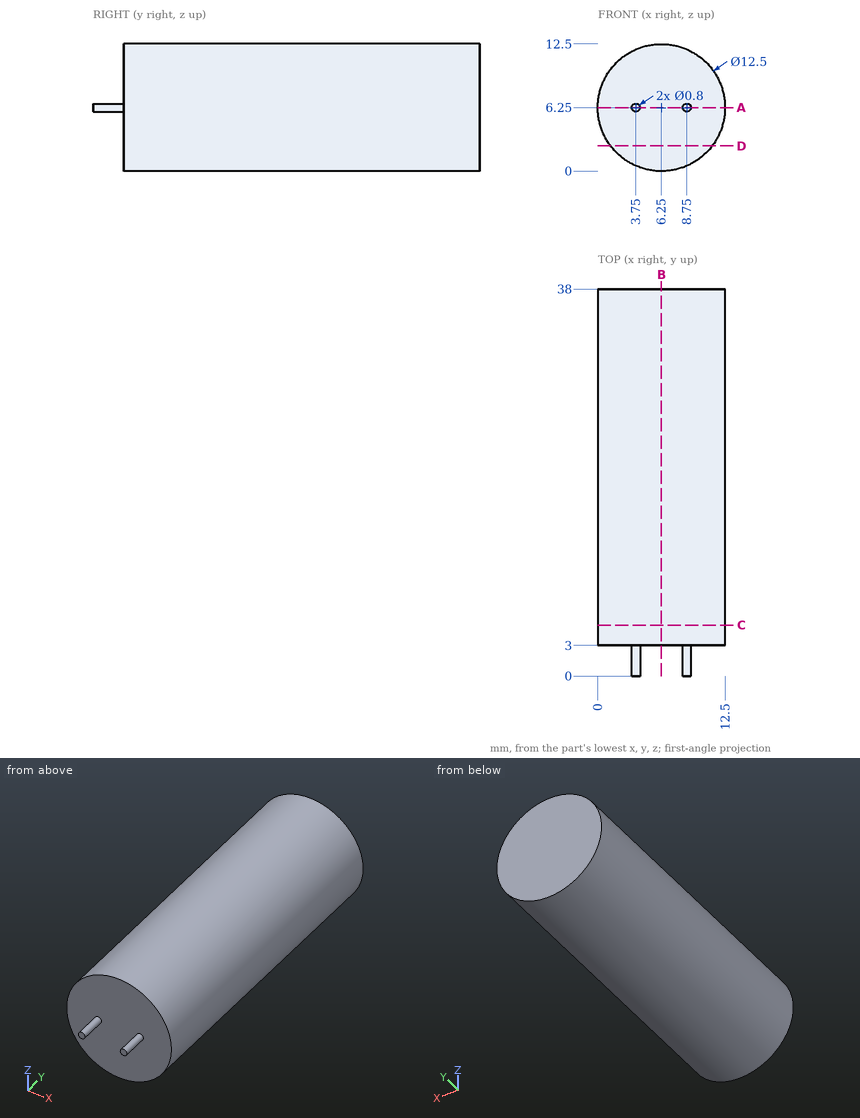
Job drawing, mm, ordinate dimensions from the low corner. One solid piece. Give positions to 0.01 mm unless a question says otherwise; leave off trailing zeros. Loops run counter-clockwise (first coordinate to the right, second up) from the corner with the lowest first, then second, coordinate; pieces in that order, holes last. Notation, with made-up numbers: (3, 4) -> (53, 4) arc R30 cw to (53, 26) -> close; hole circle Ø8 at (-33.5, 71). An arc over 180 degrees is marked (long way). Use a Markdown table: item, result. Add a question column.
(1) Slice it at C-C on y = 5. List the corners of the cut face in (x, z).
(2) Wall check: line 1 along Y through (x, z) = (9.75, 3.5); line 2 along X through (y, z) = (23, 6) (3 decimals); line 3 along X through (y, z) = (7, 0.5). Give the ranges that are in metal, low to high.
(3) Slice it at A-A on z = 6.25. List the corners of the cut face in (x, y), and give its area (3 significant figures).
(4) Slice it at B-B on x = 6.25. List the corners of the cut face in (y, z), and give its area (4 significant figures).
(5) Drop flat-ended pins along their axis: pin 1 Ø2 at (x, y) = (3.5, 9.5) entering from +Z; pin 2 Ø1 at (y, z) = (11, 3) entering from +X; pin 3 Ø2 at (x, z) = (10, 9) entering from -Y. Give the stop position or say it passes through.
(6) Slice it at D-D on z = 2.5. List the corners of the cut face in (x, y).
Filled sheet:
| question | item | result |
|---|---|---|
| 1 | outline | circle Ø12.5 at (6.25, 6.25) |
| 2 | line 1 | 3 to 38 |
| 2 | line 2 | 0.005 to 12.495 |
| 2 | line 3 | 3.8 to 8.7 |
| 3 | outline | (0, 3) -> (3.35, 3) -> (3.35, 0) -> (4.15, 0) -> (4.15, 3) -> (8.35, 3) -> (8.35, 0) -> (9.15, 0) -> (9.15, 3) -> (12.5, 3) -> (12.5, 38) -> (0, 38) -> close |
| 3 | area | 442 mm2 |
| 4 | outline | (3, 0) -> (38, 0) -> (38, 12.5) -> (3, 12.5) -> close |
| 4 | area | 437.5 mm2 |
| 5 | pin 1 | z = 12.25 |
| 5 | pin 2 | x = 11.86 |
| 5 | pin 3 | y = 3 |
| 6 | outline | (1.25, 3) -> (11.25, 3) -> (11.25, 38) -> (1.25, 38) -> close |
